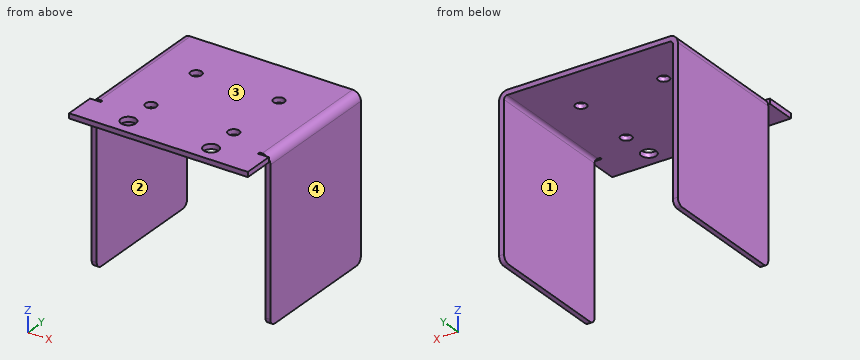
```python
from build123d import *

# Parameters (mm, degrees)
SKETCH_1_W                          = 54
SKETCH_1_H                          = 50
SM_BASE_FLANGE_1_DEPTH              = 1.5
SM_EDGE_FLANGE_1_STRIP_W            = 8
SM_EDGE_FLANGE_1_STRIP_H            = 1.5
SM_EDGE_FLANGE_1_STRIP_CUT_DEPTH    = 40
SM_EDGE_FLANGE_1_RELIEF_W           = 8.75
SM_EDGE_FLANGE_1_RELIEF_H           = 0.75
SM_EDGE_FLANGE_1_RELIEF_CUT_DEPTH   = 1.5
SM_EDGE_FLANGE_1_STRIP_2_W          = 8
SM_EDGE_FLANGE_1_STRIP_2_H          = 1.5
SM_EDGE_FLANGE_1_STRIP_CUT_2_DEPTH  = 40
SM_EDGE_FLANGE_1_RELIEF_2_W         = 8.75
SM_EDGE_FLANGE_1_RELIEF_2_H         = 0.75
SM_EDGE_FLANGE_1_RELIEF_CUT_2_DEPTH = 1.5
SM_EDGE_FLANGE_1_DEPTH              = 40
SM_EDGE_FLANGE_1_BEND_DEPTH         = 40
HOLE_WIZARD_M4_1_D                  = 4.5
HOLE_WIZARD_M4_1_2_D                = 3.3
HOLE_WIZARD_M4_1_3_D                = 3.3
OTHER_START                         = -27
OTHER_1_DEPTH                       = 54


# Read off the part's stored shape, not the designer's step: 断开-边角1
# Sheet-metal steps are written as plain solids
with BuildPart() as part:
    # Sketch 1 → 基体-法兰1 (new body)
    with BuildSketch(Plane.XY):
        Rectangle(SKETCH_1_W, SKETCH_1_H)
    extrude(amount=-SM_BASE_FLANGE_1_DEPTH)

    # 边线-法兰1 strip (across the edge) → 边线-法兰1 strip cut (cut)
    with BuildSketch(Plane(origin=(27, 25, -1.5), x_dir=(-1, 0, 0), z_dir=(0, -1, 0))):
        with Locations((-1.5, -0.75)):
            Rectangle(SM_EDGE_FLANGE_1_STRIP_W, SM_EDGE_FLANGE_1_STRIP_H)
    extrude(amount=SM_EDGE_FLANGE_1_STRIP_CUT_DEPTH, mode=Mode.SUBTRACT)

    # 边线-法兰1 relief (on the sheet) → 边线-法兰1 relief cut (cut)
    with BuildSketch(Plane(origin=(24.5, 25, -1.5), x_dir=(-1, 0, 0), z_dir=(0, 0, -1))):
        with Locations((-3.625, -40.375)):
            Rectangle(SM_EDGE_FLANGE_1_RELIEF_W, SM_EDGE_FLANGE_1_RELIEF_H)
    extrude(amount=-SM_EDGE_FLANGE_1_RELIEF_CUT_DEPTH, mode=Mode.SUBTRACT)

    # 边线-法兰1 strip 2 (across the edge) → 边线-法兰1 strip cut 2 (cut)
    with BuildSketch(Plane(origin=(-27, -15, -1.5), x_dir=(1, 0, 0), z_dir=(0, 1, 0))):
        with Locations((-1.5, -0.75)):
            Rectangle(SM_EDGE_FLANGE_1_STRIP_2_W, SM_EDGE_FLANGE_1_STRIP_2_H)
    extrude(amount=SM_EDGE_FLANGE_1_STRIP_CUT_2_DEPTH, mode=Mode.SUBTRACT)

    # 边线-法兰1 relief 2 (on the sheet) → 边线-法兰1 relief cut 2 (cut)
    with BuildSketch(Plane(origin=(-24.5, -15, -1.5), x_dir=(1, 0, 0), z_dir=(0, 0, -1))):
        with Locations((-3.625, 0.375)):
            Rectangle(SM_EDGE_FLANGE_1_RELIEF_2_W, SM_EDGE_FLANGE_1_RELIEF_2_H)
    extrude(amount=-SM_EDGE_FLANGE_1_RELIEF_CUT_2_DEPTH, mode=Mode.SUBTRACT)

    # 边线-法兰1 section (across the edge) → 边线-法兰1 (add)
    with BuildSketch(Plane(origin=(27, 25, -1.5), x_dir=(-1, 0, 0), z_dir=(0, -1, 0))):
        with BuildLine():
            Line((0, 1), (0, 47))
            Line((0, 47), (1.5, 47))
            Line((1.5, 47), (1.5, 1))
            ThreePointArc((1.5, 1), (1.792893219, 0.292893219), (2.5, 0))
            Line((2.5, 0), (2.5, -1.5))
            ThreePointArc((2.5, -1.5), (0.732233047, -0.767766953), (0, 1))
        make_face()
    extrude(amount=SM_EDGE_FLANGE_1_DEPTH)

    # 边线-法兰1 section 2 (across the edge) → 边线-法兰1 bend (add)
    with BuildSketch(Plane(origin=(-27, -15, -1.5), x_dir=(1, 0, 0), z_dir=(0, 1, 0))):
        with BuildLine():
            Line((0, 1), (0, 47))
            Line((0, 47), (1.5, 47))
            Line((1.5, 47), (1.5, 1))
            ThreePointArc((1.5, 1), (1.792893219, 0.292893219), (2.5, 0))
            Line((2.5, 0), (2.5, -1.5))
            ThreePointArc((2.5, -1.5), (0.732233047, -0.767766953), (0, 1))
        make_face()
    extrude(amount=SM_EDGE_FLANGE_1_BEND_DEPTH)

    # Hole Wizard M4 _1 (through all)
    with Locations(Plane.XY):
        with Locations((-12.5, -20), (12.5, -20)):
            Hole(HOLE_WIZARD_M4_1_D / 2)

    # Hole Wizard M4 _1 2 (through all)
    with Locations(Plane(origin=(0, 0, -1.5), x_dir=(-1, 0, 0), z_dir=(0, 0, -1))):
        with Locations((-12.5, 10), (12.5, 10)):
            Hole(HOLE_WIZARD_M4_1_2_D / 2)

    # Hole Wizard M4 _1 3 (through all)
    with Locations(Plane.XY):
        with Locations((-12.5, -10), (12.5, -10)):
            Hole(HOLE_WIZARD_M4_1_3_D / 2)

    # Other 1 outline → Other 1 (cut)
    with BuildSketch(Plane.YZ.offset(OTHER_START)):
        with BuildLine():
            Line((-15, -48.5), (-13, -48.5))
            ThreePointArc((-13, -48.5), (-14.414213562, -47.914213562), (-15, -46.5))
            Line((-15, -46.5), (-15, -48.5))
        make_face()
        with BuildLine():
            ThreePointArc((25, -46.5), (24.414213562, -47.914213562), (23, -48.5))
            Line((23, -48.5), (25, -48.5))
            Line((25, -48.5), (25, -46.5))
        make_face()
    extrude(amount=OTHER_1_DEPTH, mode=Mode.SUBTRACT)


solid = part.part
```
The listing builds one solid part. Answer for the finished solid, in the listing's coordinates (mm). Face numbers are marked on the shaded views. Give positions to 0.01 mm unless a question says otherwise; leave off trailing zeros. Order: outer loops, then holes, each group sorted by start corner. A loop starts at its lowest first (then second) coordinate and runs counter-clockwise, first axis right, second up. Notation, with made-up numbers: (-37.5, -12) -> (-20.5, -12) arc R22 cw to (-20.5, 15) -> close; hole circle Ø11 at (32, 60). An arc over 180 degrees is marked (long way). Answer as a JSON object with one key per item and string values. Group by question number.
Item 1: Flat-ended cylindrical pins translate along their axes: pin 1 (2.5 mm diameter, centred on x = 12.5, y = -20, fed in from -Z); pin 2 (6 mm diameter, centred on x = 7.5, y = -19, fed in from -Z); pin 3 (1.6 mm diameter, centred on x = 25, z = -24, fed in from -Y). Find the tip coordinate at first contact, or state that the pin passes through.
Item 2: The part is cut by section D-D on y = -2. Write down the section's boundary in (x, z), and give its area (3 significant figures).
Item 3: Consider L1, parallel to Y at x = 12.5, z = -1.1; L2, parallel to X at y = 7.5, z = -27; L3, parallel to Z at x = 16, y = 0.5. Determine where each line is inside the solid, lowest interval first. Write a range as from..to.
Item 4: The part is cut by section B-B on x = -12.5. Write down the section's boundary in (y, z).
Item 5: Determine the mould class of the marked faces 1, 2, 3 and 4 for opening direction X: pulls with the +X half, pulls with the -X half, needs draft (parallel to the pull), parting line crosses it, or undercut.
Item 6: The part is cut by section C-C on z = -30. Write down the section's boundary in (x, y), and give its area (3 significant figures).
Item 7: The part is cut by section A-A on y = -10. Write down the section's boundary in (x, z).
Result set:
{
 "1": {"pin 1": "through", "pin 2": "z = -1.5", "pin 3": "y = -15"},
 "2": {"outline": "(-27, -48.5) -> (-25.5, -48.5) -> (-25.5, -2.5) arc R1 cw to (-24.5, -1.5) -> (24.5, -1.5) arc R1 cw to (25.5, -2.5) -> (25.5, -48.5) -> (27, -48.5) -> (27, -2.5) arc R2.5 ccw to (24.5, 0) -> (-24.5, 0) arc R2.5 ccw to (-27, -2.5) -> close", "area": "220 mm²"},
 "3": {"L1": "-25..-22.25, -17.75..-11.65, -8.35..8.35, 11.65..25", "L2": "-27..-25.5, 25.5..27", "L3": "-1.5..0"},
 "4": {"outline": "(-25, -1.5) -> (-22.25, -1.5) -> (-22.25, 0) -> (-25, 0) -> close; (-17.75, -1.5) -> (-11.65, -1.5) -> (-11.65, 0) -> (-17.75, 0) -> close; (-8.35, -1.5) -> (8.35, -1.5) -> (8.35, 0) -> (-8.35, 0) -> close; (11.65, -1.5) -> (25, -1.5) -> (25, 0) -> (11.65, 0) -> close"},
 "5": {"face 1": "undercut", "face 2": "undercut", "face 3": "needs draft", "face 4": "pulls with the +X half"},
 "6": {"outline": "(-27, -15) -> (-25.5, -15) -> (-25.5, 25) -> (-27, 25) -> close; (25.5, -15) -> (27, -15) -> (27, 25) -> (25.5, 25) -> close", "area": "120 mm²"},
 "7": {"outline": "(-27, -48.5) -> (-25.5, -48.5) -> (-25.5, -2.5) arc R1 cw to (-24.5, -1.5) -> (-14.15, -1.5) -> (-14.15, 0) -> (-24.5, 0) arc R2.5 ccw to (-27, -2.5) -> close; (-10.85, -1.5) -> (10.85, -1.5) -> (10.85, 0) -> (-10.85, 0) -> close; (14.15, -1.5) -> (24.5, -1.5) arc R1 cw to (25.5, -2.5) -> (25.5, -48.5) -> (27, -48.5) -> (27, -2.5) arc R2.5 ccw to (24.5, 0) -> (14.15, 0) -> close"}
}
